Source: CAD feature listing. Evaluate the final solid. Frame: model axes, mm. Coordinates: 2 decimals unless noted, no trailing zeros. Loops run counter-clockwise (first coordinate to the right, second up) from the corner with the lowest first, then second, coordinate; pieces in that order, holes last.
```python
from build123d import *

# Parameters (mm, degrees)
SKETCH1_W           = 317.5
SKETCH1_H           = 38.1
BOSS_EXTRUDE1_DEPTH = 4.7625
SKETCH2_R           = 4.4196
SKETCH2_R_2         = 6.477
SKETCH2_R_3         = 2.19075
CUT_EXTRUDE1_DEPTH  = 161.172377846
SKETCH3_R           = 1.5113
CUT_EXTRUDE2_DEPTH  = 161.172377846
FILLET1_R           = 2.54
SKETCH4_R           = 8.73125
CUT_EXTRUDE3_DEPTH  = 161.172377846


with BuildPart() as part:
    # Sketch1 → Boss-Extrude1 (new, symmetric)
    with BuildSketch(Plane(origin=(0, 0, 0), x_dir=(1, 0, 0), z_dir=(0, 1, 0))):
        Rectangle(SKETCH1_W, SKETCH1_H)
    extrude(amount=BOSS_EXTRUDE1_DEPTH, both=True)

    # Sketch2 → Cut-Extrude1 (cut, through all)
    with BuildSketch(Plane(origin=(0, 4.7625, 0), x_dir=(1, 0, 0), z_dir=(0, 1, 0))):
        with Locations(Location((-99.06, 0, 0), (0, 0, 270))):
            Circle(SKETCH2_R)
        with Locations(Location((-57.15, 0, 0), (0, 0, 270))):
            Circle(SKETCH2_R)
        with Locations(Location((-19.05, 0, 0), (0, 0, 270))):
            Circle(SKETCH2_R)
        with Locations(Location((19.05, 0, 0), (0, 0, 270))):
            Circle(SKETCH2_R)
        with Locations(Location((57.15, 0, 0), (0, 0, 270))):
            Circle(SKETCH2_R)
        with Locations(Location((-142.24, 0, 0), (0, 0, 270))):
            Circle(SKETCH2_R_2)
        with Locations(Location((-142.24, -10.31875, 0), (0, 0, 270))):
            Circle(SKETCH2_R_3)
        with Locations(Location((-142.24, 10.31875, 0), (0, 0, 270))):
            Circle(SKETCH2_R_3)
        with Locations(Location((142.24, 0, 0), (0, 0, 270))):
            Circle(SKETCH2_R_2)
        with Locations(Location((142.24, -10.31875, 0), (0, 0, 270))):
            Circle(SKETCH2_R_3)
        with Locations(Location((142.24, 10.31875, 0), (0, 0, 270))):
            Circle(SKETCH2_R_3)
        with Locations(Location((99.06, 0, 0), (0, 0, 270))):
            Circle(SKETCH2_R)
    extrude(amount=-CUT_EXTRUDE1_DEPTH, mode=Mode.SUBTRACT)

    # Sketch3 → Cut-Extrude2 (cut, through all)
    with BuildSketch(Plane(origin=(0, 4.7625, 0), x_dir=(1, 0, 0), z_dir=(0, 1, 0))):
        with Locations(Location((-154.94, 15.24, 0), (0, 0, 270))):
            Circle(SKETCH3_R)
        with Locations(Location((-154.94, -15.24, 0), (0, 0, 270))):
            Circle(SKETCH3_R)
        with Locations(Location((154.94, -15.24, 0), (0, 0, 270))):
            Circle(SKETCH3_R)
        with Locations(Location((154.94, 15.24, 0), (0, 0, 270))):
            Circle(SKETCH3_R)
        with Locations(Location((0, 15.24, 0), (0, 0, 270))):
            Circle(SKETCH3_R)
        with Locations(Location((0, -15.24, 0), (0, 0, 270))):
            Circle(SKETCH3_R)
    extrude(amount=-CUT_EXTRUDE2_DEPTH, mode=Mode.SUBTRACT)

    # Fillet1
    fillet1_edges = [part.edges().sort_by_distance(p)[0] for p in [
        (158.75, 0, 19.05),
        (-158.75, 0, 19.05),
        (-158.75, 0, -19.05),
        (158.75, 0, -19.05),
    ]]
    fillet(fillet1_edges, radius=FILLET1_R)

    # Sketch4 → Cut-Extrude3 (cut, through all)
    with BuildSketch(Plane(origin=(0, 4.7625, 0), x_dir=(1, 0, 0), z_dir=(0, 1, 0))):
        with Locations(Location((99.06, 0, 0), (0, 0, 270))):
            Circle(SKETCH4_R)
        with Locations(Location((-99.06, 0, 0), (0, 0, 270))):
            Circle(SKETCH4_R)
        with Locations(Location((-57.15, 0, 0), (0, 0, 270))):
            Circle(SKETCH4_R)
        with Locations(Location((-19.05, 0, 0), (0, 0, 270))):
            Circle(SKETCH4_R)
        with Locations(Location((19.05, 0, 0), (0, 0, 270))):
            Circle(SKETCH4_R)
        with Locations(Location((57.15, 0, 0), (0, 0, 270))):
            Circle(SKETCH4_R)
    extrude(amount=-CUT_EXTRUDE3_DEPTH, mode=Mode.SUBTRACT)


solid = part.part
```
Q1. Draft query along Z for faces 1 (the flat face through (-2, 0, -19.05)), 2 (the cylindrical face through (148.662, 0.067, -0.843)), 3 (the flat face through (-2, -4.762, 0)). Return one class per face: released by +Z, released by -Z, zero draft, split by the parting line, or undercut.
Q2. Section query D-D on x = 51. Return the cut outline in (y, z), then the cut area to 3 significant figures.
Q3. Section query A-A on x = -57.15. Return the cut outline in (y, z), then the cut area to 3 significant figures.
Q4. Material intervals for line 1 along X through (y, z) = (0, -15.24); line 2 along X through (y, z) = (-0.75, 10.5); line 3 along X through (y, z) = (0.75, -11), sorted ascending.
Q5. Section query B-B on y = 1. Count the separate pieces of the cut face and the enclosed holes in it, then the cut area to 3 significant figures.
Resolved:
1. face 1: released by -Z
1. face 2: undercut
1. face 3: zero draft
2. outline: (-4.76, -19.05) - (4.76, -19.05) - (4.76, -6.2) - (-4.76, -6.2) - close; (-4.76, 6.2) - (4.76, 6.2) - (4.76, 19.05) - (-4.76, 19.05) - close
2. area: 245 mm2
3. outline: (-4.76, -19.05) - (4.76, -19.05) - (4.76, -8.73) - (-4.76, -8.73) - close; (-4.76, 8.73) - (4.76, 8.73) - (4.76, 19.05) - (-4.76, 19.05) - close
3. area: 197 mm2
4. line 1: x = -158.75 to -156.45, -153.43 to -1.51, 1.51 to 153.43, 156.45 to 158.75
4. line 2: x = -158.75 to -144.42, -140.06 to 140.06, 144.42 to 158.75
4. line 3: x = -158.75 to -144.32, -140.16 to 140.16, 144.32 to 158.75
5. separate pieces: 1
5. enclosed holes: 18
5. area: 10,300 mm2
